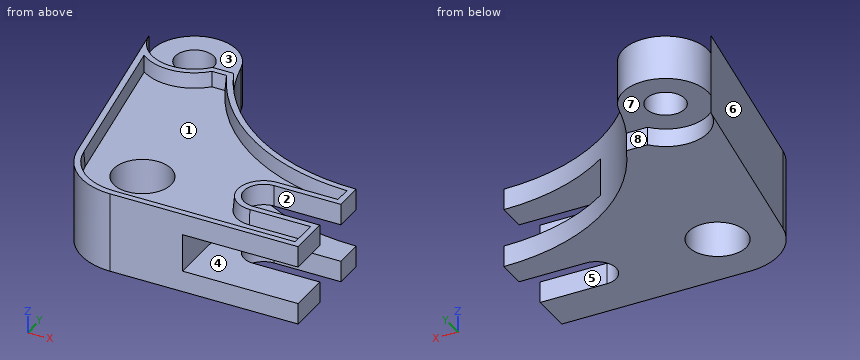
```python
from build123d import *

# Parameters (mm, degrees)
SKETCH2_R               = 6.35
SKETCH2_R_2             = 9.5
BOSS_EXTRUDE2_DEPTH     = 26.5
CUT_EXTRUDE1_START      = -6
CUT_EXTRUDE1_DEPTH      = 6
CUT_EXTRUDE2_DEPTH      = 6
CUT_EXTRUDE3_DEPTH      = 6.25
CUT_EXTRUDE3_DEPTH_BACK = 6.25
CUT_EXTRUDE7_DEPTH      = 5
CUT_EXTRUDE7_DRAFT      = -5


with BuildPart() as part:
    # Sketch2 → Boss-Extrude2 (new body)
    with BuildSketch(Plane.XY):
        with BuildLine():
            Line((0, 0), (-62, 0))
            ThreePointArc((-62, 0), (-74.874173195, 4.694587084), (-81.704453671, 16.574433546))
            Line((-81.704453671, 16.574433546), (-93.133993592, 82.319133844))
            ThreePointArc((-93.133993592, 82.319133844), (-82.120785811, 98.438258498), (-65.702115422, 87.876810306))
            ThreePointArc((-65.702115422, 87.876810306), (-41.950384105, 50.414084566), (0, 36))
            Line((0, 36), (0, 26.5))
            Line((0, 26.5), (-22, 26.5))
            ThreePointArc((-22, 26.5), (-28.5, 20), (-22, 13.5))
            Line((-22, 13.5), (0, 13.5))
            Line((0, 13.5), (0, 0))
        make_face()
        with Locations((-79.340876022, 84.717030361)):
            Circle(SKETCH2_R, mode=Mode.SUBTRACT)
        with Locations((-62, 20)):
            Circle(SKETCH2_R_2, mode=Mode.SUBTRACT)
    extrude(amount=BOSS_EXTRUDE2_DEPTH)

    # Sketch3 → Cut-Extrude1 (cut)
    with BuildSketch(Plane.XY.offset(26.5).offset(CUT_EXTRUDE1_START)):
        with BuildLine():
            Line((-68.617070727, 75.717030361), (-61.624981931, 75.717030361))
            ThreePointArc((-61.624981931, 75.717030361), (-63.955170346, 81.699140564), (-65.702115422, 87.876810306))
            ThreePointArc((-65.702115422, 87.876810306), (-92.955159562, 87.980660806), (-68.617070727, 75.717030361))
        make_face()
    extrude(amount=CUT_EXTRUDE1_DEPTH, mode=Mode.SUBTRACT)

    # Sketch4 → Cut-Extrude2 (cut)
    with BuildSketch(Plane(origin=(0, 0, 0), x_dir=(-1, 0, 0), z_dir=(0, 0, -1))):
        with BuildLine():
            Line((68.617070727, 75.717030361), (61.624981931, 75.717030361))
            ThreePointArc((61.624981931, 75.717030361), (63.955170346, 81.699140564), (65.702115422, 87.876810306))
            ThreePointArc((65.702115422, 87.876810306), (92.955159562, 87.980660806), (68.617070727, 75.717030361))
        make_face()
    extrude(amount=-CUT_EXTRUDE2_DEPTH, mode=Mode.SUBTRACT)

    # Sketch6 → Cut-Extrude3 (cut, two sides: drawn at the far end of the back side and taken through both)
    with BuildSketch(Plane.XY.offset(13.25).offset(-CUT_EXTRUDE3_DEPTH_BACK)):
        with BuildLine():
            Line((0, 0), (-38.108793453, 0))
            Line((-38.108793453, 0), (-38.108793453, 47.596659083))
            ThreePointArc((-38.108793453, 47.596659083), (-19.936162439, 38.900682282), (0, 36))
            Line((0, 36), (0, 0))
        make_face()
    extrude(amount=CUT_EXTRUDE3_DEPTH + CUT_EXTRUDE3_DEPTH_BACK, mode=Mode.SUBTRACT)


with BuildPart() as cut_extrude7_tool:
    # Sketch7 → Cut-Extrude7 (with draft: the straight prism first)
    with BuildSketch(Plane.XY.offset(26.5)):
        with BuildLine():
            Line((-89.350908837, 72.235073662), (-79.734008304, 16.916990192))
            ThreePointArc((-79.734008304, 16.916990192), (-73.586755876, 6.225128375), (-62, 2))
            Line((-62, 2), (-2, 2))
            Line((-2, 2), (-2, 11.5))
            Line((-2, 11.5), (-22, 11.5))
            ThreePointArc((-22, 11.5), (-30.5, 20), (-22, 28.5))
            Line((-22, 28.5), (-2, 28.5))
            Line((-2, 28.5), (-2, 34.016457666))
            ThreePointArc((-2, 34.016457666), (-38.108007625, 45.193460051), (-62.909611076, 73.717030361))
            Line((-62.909611076, 73.717030361), (-67.721925983, 73.717030361))
            ThreePointArc((-67.721925983, 73.717030361), (-78.247165561, 68.754455462), (-89.350908837, 72.235073662))
        make_face()
    extrude(amount=-CUT_EXTRUDE7_DEPTH)
    # Cut-Extrude7: the draft: its side faces are tilted about the plane it starts from
    cut_extrude7_sides = [cut_extrude7_tool.faces().sort_by_distance(p)[0] for p in [
        (-38.108007625, 45.193460051, 24),
        (-65.31576853, 73.717030361, 24),
        (-78.247165561, 68.754455462, 24),
        (-84.542458571, 44.576031927, 24),
        (-73.586755876, 6.225128375, 24),
        (-32, 2, 24),
        (-2, 6.75, 24),
        (-12, 11.5, 24),
        (-30.5, 20, 24),
        (-12, 28.5, 24),
        (-2, 31.258228833, 24),
    ]]
    draft(cut_extrude7_sides, Plane.XY.offset(26.5), CUT_EXTRUDE7_DRAFT)


with BuildPart() as part_1:
    add(part.part)

    # Cut-Extrude7: cut by cut_extrude7_tool
    add(cut_extrude7_tool.part, mode=Mode.SUBTRACT)


solid = part_1.part
```
Verification items for the finished model (mm, model axes). Face numbers are marked on the shaded views. A direction names the side the tool comes from. Coordinates: 2 decimals unless noted, no trailing zeros. Order: outer loops, then holes, each group sorted by start corner. A loop starts at its lowest first (then second) coordinate and runs counter-clockwise, first axis right, second up. Notation, with made-up numbers: (29, 17.25) - (59, 17.25) arc R36 ccw to (59, 56.25) - close; hole circle Ø7 at (-33.75, 52.5). An arc over 180 degrees is marked (long way). Return JSON: item names as keys, results as strings.
(1) Thickness scan on line 1 along Z through (x, y) = (-33, 35.5); line 2 along Z through (x, y) = (-69.5, 12); line 3 along Y through (x, z) = (-62, 9.5). Record the ranges inside material, lowest first.
Filled sheet:
{"line 1": "z = 0 to 7, 19.5 to 21.5", "line 2": "z = 0 to 21.5", "line 3": "y = 0 to 10.5, 29.5 to 76.57"}
(2) Mould release check, pull along Y, two halves, no side actions. Record for the marked faces 5, 6, 7 and 8: pulls with the +Y half, pulls with the -Y half, needs draft (parallel to the pull), parting line crosses it, or undercut.
Filled sheet:
{"face 5": "undercut", "face 6": "pulls with the -Y half", "face 7": "needs draft", "face 8": "pulls with the +Y half"}
(3) Section check D-D, the plane x = -25. Give the number of separate pieces and of enclosed holes in the cut face, and give its area (3 significant figures).
Filled sheet:
{"separate pieces": "4", "enclosed holes": "0", "area": "309 mm^2"}
(4) Go/stop test with flat-tipped pins: pin 1 (3 mm diameter, centred on x = -19.5, z = 17, fed in from -Y); pin 2 (3.5 mm diameter, centred on x = -12.5, z = 24, fed in from +Y); pin 3 (1.5 mm diameter, centred on x = -20.5, z = 3.5, fed in from +Y); pin 4 (14 mm diameter, centred on x = -77.5, y = 79, fed in from +Z). Record where each tip stops, or that it passes through.
Filled sheet:
{"pin 1": "passes through", "pin 2": "stops at y = 37.44", "pin 3": "stops at y = 39.32", "pin 4": "stops at z = 20.5"}
(5) Section check B-B, the plane y = 20. Record the cut outline in (x, z).
Filled sheet:
{"outline": "(-82.3, 0) - (-71.5, 0) - (-71.5, 21.5) - (-79.83, 21.5) - (-80.27, 26.5) - (-82.3, 26.5) - close; (-52.5, 0) - (-28.5, 0) - (-28.5, 7) - (-38.11, 7) - (-38.11, 19.5) - (-28.5, 19.5) - (-28.5, 26.5) - (-30.5, 26.5) - (-30.94, 21.5) - (-52.5, 21.5) - close"}
(6) Section check C-C, the plane z = 13. Record the cut outline in (x, y).
Filled sheet:
{"outline": "(-93.13, 82.32) - (-81.7, 16.57) arc R20 ccw to (-62, 0) - (-38.11, 0) - (-38.11, 47.6) arc R67 cw to (-65.7, 87.88) arc R14 ccw to start; hole circle Ø12.7 at (-79.34, 84.72); hole circle Ø19 at (-62, 20)"}
(7) Access from +Z, -Z, +X, -X, +Y, -Y to the whole of each face (thin tool, end or side, straight path). Record for the marked faces 1, 2, 3 and 4.
Filled sheet:
{"face 1": "+Z", "face 2": "+Z, -Z, +X", "face 3": "+Z, +Y", "face 4": "+X, +Y, -Y"}
(8) Section check A-A, the plane z = 4.25. Record the cut outline in (x, y).
Filled sheet:
{"outline": "(-93.13, 82.32) - (-81.7, 16.57) arc R20 ccw to (-62, 0) - (0, 0) - (0, 13.5) - (-22, 13.5) arc R6.5 cw to (-22, 26.5) - (0, 26.5) - (0, 36) arc R67 cw to (-61.62, 75.72) - (-68.62, 75.72) arc R14 cw to start; hole circle Ø19 at (-62, 20)"}
